Design review of the part built by this model. Coordinates are the model's own, in mm. Give positions to 0.01 mm unless a question says otherwise; leave off trailing zeros. Write each loop counter-clockwise with the first axis right and the second up, starting at its lowest first coordinate (ties: lowest second). Pieces come first, ordered by that corner, then holes. Notation, with made-up numbers: M 52,-20 L 79,-20 A10 ccw 79,-2 Z; hole C 3.25,10.5 d11. An arc over 180 degrees is marked long. Use one line per item in the form item = value. Start each with the question number.
from build123d import *

# Parameters (mm, degrees)
CROQUIS1_R              = 25
SALIENTE_EXTRUIR1_DEPTH = 35
CROQUIS2_R              = 50
SALIENTE_EXTRUIR2_DEPTH = 20
CORTAR_EXTRUIR1_REACH   = 116.455
CROQUIS3_R              = 5


with BuildPart() as part:
    # Croquis1 → Saliente-Extruir1 (new, symmetric)
    with BuildSketch(Plane(origin=(0, 0, 0), x_dir=(1, 0, 0), z_dir=(0, 1, 0))):
        with Locations(Location((0, 0, 0), (0, 0, 270))):
            Circle(CROQUIS1_R)
    extrude(amount=SALIENTE_EXTRUIR1_DEPTH, both=True)

    # Croquis2 → Saliente-Extruir2 (add)
    with BuildSketch(Plane(origin=(0, 35, 0), x_dir=(1, 0, 0), z_dir=(0, 1, 0))):
        with Locations(Location((0, 0, 0), (0, 0, 270))):
            Circle(CROQUIS2_R)
    extrude(amount=SALIENTE_EXTRUIR2_DEPTH)

    # Croquis3 → Cortar-Extruir1 (cut, up to next)
    with BuildSketch(Plane(origin=(0, 55, 0), x_dir=(1, 0, 0), z_dir=(0, 1, 0)), mode=Mode.PRIVATE) as cortar_extruir1_sk1:
        with Locations(Location((0, 37.5, 0), (0, 0, 270))):
            Circle(CROQUIS3_R)
    cortar_extruir1_tool1 = extrude(cortar_extruir1_sk1.sketch, amount=-CORTAR_EXTRUIR1_REACH, mode=Mode.PRIVATE) & part.part
    # Croquis3 → Cortar-Extruir1 (cut, up to next)
    with BuildSketch(Plane(origin=(0, 55, 0), x_dir=(1, 0, 0), z_dir=(0, 1, 0)), mode=Mode.PRIVATE) as cortar_extruir1_sk2:
        with Locations(Location((37.5, 0, 0), (0, 0, 270))):
            Circle(CROQUIS3_R)
    cortar_extruir1_tool2 = extrude(cortar_extruir1_sk2.sketch, amount=-CORTAR_EXTRUIR1_REACH, mode=Mode.PRIVATE) & part.part
    # Croquis3 → Cortar-Extruir1 (cut, up to next)
    with BuildSketch(Plane(origin=(0, 55, 0), x_dir=(1, 0, 0), z_dir=(0, 1, 0)), mode=Mode.PRIVATE) as cortar_extruir1_sk3:
        with Locations(Location((0, -37.5, 0), (0, 0, 270))):
            Circle(CROQUIS3_R)
    cortar_extruir1_tool3 = extrude(cortar_extruir1_sk3.sketch, amount=-CORTAR_EXTRUIR1_REACH, mode=Mode.PRIVATE) & part.part
    # Croquis3 → Cortar-Extruir1 (cut, up to next)
    with BuildSketch(Plane(origin=(0, 55, 0), x_dir=(1, 0, 0), z_dir=(0, 1, 0)), mode=Mode.PRIVATE) as cortar_extruir1_sk4:
        with Locations(Location((-37.5, 0, 0), (0, 0, 270))):
            Circle(CROQUIS3_R)
    cortar_extruir1_tool4 = extrude(cortar_extruir1_sk4.sketch, amount=-CORTAR_EXTRUIR1_REACH, mode=Mode.PRIVATE) & part.part
    add(cortar_extruir1_tool1.solids().sort_by_distance((0, 55, -37.5))[0], mode=Mode.SUBTRACT)
    add(cortar_extruir1_tool2.solids().sort_by_distance((37.5, 55, 0))[0], mode=Mode.SUBTRACT)
    add(cortar_extruir1_tool3.solids().sort_by_distance((0, 55, 37.5))[0], mode=Mode.SUBTRACT)
    add(cortar_extruir1_tool4.solids().sort_by_distance((-37.5, 55, 0))[0], mode=Mode.SUBTRACT)


solid = part.part
1. We need section B-B (y = 39.5). State the section outline as (x, z) points.
2. We need section C-C (x = 37.5). State the section outline as (y, z) points.
3. Draft analysis for pull direction Z (two halves, no side actions). For faces 1 (the cylindrical face through (0.22, 45.14, -42.495)), 2 (the flat face through (22.9, 35, 10.4)), 3 (the cylindrical face through (7.509, 0.49, 23.846)), 4 (the cylindrical face through (-32.543, 45.14, -0.651)), state which applies: pulls with the +Z half, pulls with the -Z half, needs draft (parallel to the pull), parting line crosses it, or undercut.
4. Clearance check with flat-ended pins moving along their axes: pin 1 Ø1.5 at (x, y) = (10.5, 3) entering from -Z; pin 2 Ø4 at (y, z) = (39, 14.5) entering from -X; pin 3 Ø12 at (y, z) = (32.5, -31) entering from +X. State where each tip first meets the part, or that it passes through.
5. To check wall thickness, follow L1, parallel to X at y = 49, z = 0; L2, parallel to Y at x = 24, z = -32.5; L3, parallel to Z at x = -1, y = 46.5. State the ranges of each line that lie inside material, in increasing order.
6. We need section D-D (z = -34.5). State the section outline as (x, y) points.
7. We need section A-A (z = 0). State the section outline as (x, y) points.
Answer block:
q1.outline = C 0,0 d100; hole C -37.5,0 d10; hole C 0,-37.5 d10; hole C 0,37.5 d10; hole C 37.5,0 d10
q2.outline = M 35,-33.07 L 55,-33.07 L 55,-5 L 35,-5 Z; M 35,5 L 55,5 L 55,33.07 L 35,33.07 Z
q3.face_1 = undercut
q3.face_2 = needs draft
q3.face_3 = parting line crosses it
q3.face_4 = undercut
q4.pin_1 = -23.02
q4.pin_2 = -48.41
q4.pin_3 = 42.98
q5.L1 = -50 to -42.5, -32.5 to 32.5, 42.5 to 50
q5.L2 = 35 to 55
q5.L3 = -49.99 to -42.4, -32.6 to 32.6, 42.4 to 49.99
q6.outline = M -36.19,35 L -4,35 L -4,55 L -36.19,55 Z; M 4,35 L 36.19,35 L 36.19,55 L 4,55 Z
q7.outline = M -50,35 L -42.5,35 L -42.5,55 L -50,55 Z; M -32.5,35 L -25,35 L -25,-35 L 25,-35 L 25,35 L 32.5,35 L 32.5,55 L -32.5,55 Z; M 42.5,35 L 50,35 L 50,55 L 42.5,55 Z
